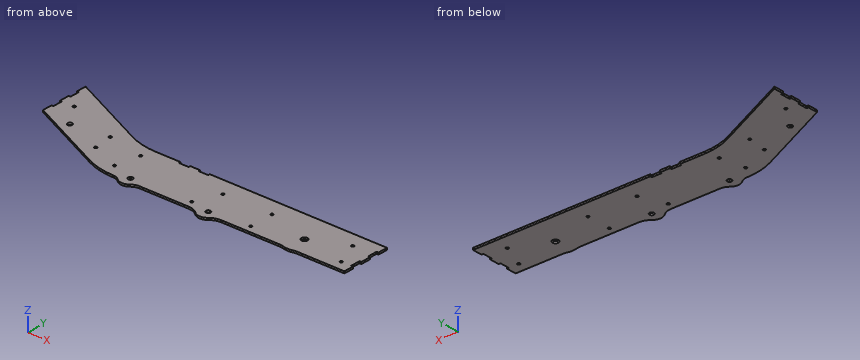
from build123d import *

# Parameters (mm, degrees)
BOSS_EXTRUDE1_DEPTH              = 4.826
SKETCH5_R                        = 3.3782
STANDOFF_HOLE_DEPTH              = 5.826
SKETCH8_W                        = 25.4
SKETCH8_H                        = 4.826
TOP_SLOTS_DEPTH                  = 5.826
BACK_AXLE_EXTENSION_DEPTH        = 4.826
LOWER_SMALL_AXLE_EXTENSION_DEPTH = 4.826
FRONT_SMALL_AXLE_EXTENSION_DEPTH = 4.826
SKETCH10_R                       = 8
SKETCH10_R_2                     = 6
NEW_AXLE_HOLES_DEPTH             = 5.826


with BuildPart() as part:
    # outer face → Boss-Extrude1 (new body)
    with BuildSketch(Plane.XY):
        with BuildLine():
            Line((622.3, 0), (24.193267589, 0))
            ThreePointArc((24.193267589, 0), (-14.28969577, 4.214569934), (-50.948259349, 16.658475465))
            Line((-50.948259349, 16.658475465), (-254, 111.343057132))
            Line((-254, 111.343057132), (-254, 136.743057132))
            Line((-254, 136.743057132), (-249.174, 136.743057132))
            Line((-249.174, 136.743057132), (-249.174, 162.143057132))
            Line((-249.174, 162.143057132), (-254, 162.143057132))
            Line((-254, 162.143057132), (-254, 187.543057132))
            Line((-254, 187.543057132), (-249.174, 187.543057132))
            Line((-249.174, 187.543057132), (-249.174, 212.943057132))
            Line((-249.174, 212.943057132), (-254, 212.943057132))
            Line((-254, 212.943057132), (-254, 238.343057132))
            Line((-254, 238.343057132), (-50.948259349, 143.658475465))
            ThreePointArc((-50.948259349, 143.658475465), (-14.28969577, 131.214569934), (24.193267589, 127))
            Line((24.193267589, 127), (622.3, 127))
            Line((622.3, 127), (622.3, 101.6))
            Line((622.3, 101.6), (617.474, 101.6))
            Line((617.474, 101.6), (617.474, 76.2))
            Line((617.474, 76.2), (622.3, 76.2))
            Line((622.3, 76.2), (622.3, 50.8))
            Line((622.3, 50.8), (617.474, 50.8))
            Line((617.474, 50.8), (617.474, 25.4))
            Line((617.474, 25.4), (622.3, 25.4))
            Line((622.3, 25.4), (622.3, 0))
        make_face()
    extrude(amount=BOSS_EXTRUDE1_DEPTH)

    # Sketch5 → standoff hole (cut, through all)
    with BuildSketch(Plane.XY.offset(4.826)):
        with Locations((-76.2, 63.5)):
            Circle(SKETCH5_R)
        with Locations((-82.55, 114.3)):
            Circle(SKETCH5_R)
        with Locations((592.074, 25.4)):
            Circle(SKETCH5_R)
        with Locations((0, 31.75)):
            Circle(SKETCH5_R)
        with Locations((211.0486, 19.05)):
            Circle(SKETCH5_R)
        with Locations((236.4486, 82.55)):
            Circle(SKETCH5_R)
        with Locations((363.4486, 82.55)):
            Circle(SKETCH5_R)
        with Locations((363.4486, 19.05)):
            Circle(SKETCH5_R)
        with Locations((566.674, 88.9)):
            Circle(SKETCH5_R)
        with Locations((12.7, 95.25)):
            Circle(SKETCH5_R)
        with Locations((-217.424, 162.143057132)):
            Circle(SKETCH5_R)
    extrude(amount=-STANDOFF_HOLE_DEPTH, mode=Mode.SUBTRACT)

    # Sketch8 → top slots (cut, through all)
    with BuildSketch(Plane.XY.offset(4.826)):
        with Locations((100.393267589, 124.587)):
            Rectangle(SKETCH8_W, SKETCH8_H)
        with Locations((151.193267589, 124.587)):
            Rectangle(SKETCH8_W, SKETCH8_H)
    extrude(amount=-TOP_SLOTS_DEPTH, mode=Mode.SUBTRACT)

    # Sketch9 → back axle extension (add)
    with BuildSketch(Plane.XY.offset(4.826)):
        with BuildLine():
            Line((498.944734517, 0), (456.603265483, 0))
            ThreePointArc((456.603265483, 0), (460.166971419, -0.251242575), (463.660176989, -1))
            ThreePointArc((463.660176989, -1), (477.774, -3), (491.887823011, -1))
            ThreePointArc((491.887823011, -1), (495.381028581, -0.251242575), (498.944734517, 0))
        make_face()
    extrude(amount=-BACK_AXLE_EXTENSION_DEPTH)

    # Sketch11 → lower small axle extension (add)
    with BuildSketch(Plane.XY.offset(4.826)):
        with BuildLine():
            Line((303.790106689, 0), (219.957893311, 0))
            ThreePointArc((219.957893311, 0), (233.396420016, -2.448688664), (245.107557324, -9.48))
            ThreePointArc((245.107557324, -9.48), (261.874, -15.8), (278.640442676, -9.48))
            ThreePointArc((278.640442676, -9.48), (290.351579984, -2.448688664), (303.790106689, 0))
        make_face()
    extrude(amount=-LOWER_SMALL_AXLE_EXTENSION_DEPTH)

    # Sketch13 → front small axle extension (add)
    with BuildSketch(Plane.XY.offset(4.826)):
        with BuildLine():
            Line((91.928424908, 0), (24.193267589, 0))
            ThreePointArc((24.193267589, 0), (33.393269649, -1.659006827), (41.434305199, -6.427034599))
            ThreePointArc((41.434305199, -6.427034599), (58.060846248, -12.625), (74.687387297, -6.427034599))
            ThreePointArc((74.687387297, -6.427034599), (82.728422848, -1.659006827), (91.928424908, 0))
        make_face()
    extrude(amount=-FRONT_SMALL_AXLE_EXTENSION_DEPTH)

    # Sketch10 → new axle holes (cut, through all)
    with BuildSketch(Plane.XY.offset(4.826)):
        with Locations((477.774, 47.8)):
            Circle(SKETCH10_R)
        with Locations((261.874, 9.6)):
            Circle(SKETCH10_R_2)
        with Locations((58.060846248, 12.775)):
            Circle(SKETCH10_R_2)
        with Locations((-176.843107922, 102.547565902)):
            Circle(SKETCH10_R_2)
    extrude(amount=-NEW_AXLE_HOLES_DEPTH, mode=Mode.SUBTRACT)


solid = part.part
Model file for the job. Use its own axes, mm. Round coordinates to 2 decimals unless told otherwise and drop trailing zeros. Order: outer loops, then holes, each group sorted by start corner. A loop starts at its lowest first (then second) coordinate and runs counter-clockwise, first axis right, second up.
(1) Band-saw the part on A-A (x = 513.5). List the corners of the cut face in (y, z), then the cut area to 3 significant figures.
(2) Drill centre lines: line 1 (Y direction, x = 303, z = 3.4); line 2 (Y direction, x = 496, z = 0.95); line 3 (Y direction, x = 0, z = 3.6). Where is each one in solid material? Low to high.
(3) Pin check, flat tips, straight feed: pin 1 (1.4 mm diameter, centred on x = -251, z = 2.5, fed in from -Y); pin 2 (4 mm diameter, centred on x = 12.7, y = 95.25, fed in from -Z); pin 3 (1 mm diameter, centred on x = 130.5, z = 2, fed in from -Y); pin 4 (1.4 mm diameter, centred on x = 620.5, z = 2.5, fed in from +Y). Stop position of each tip, or through.
(4) Band-saw the part on B-B (z = 1.45). Give the number of separate pieces and of enclosed holes in the cut face, then the cut area to 3 significant figures.
Verdict:
1. outline: (0, 0) - (127, 0) - (127, 4.83) - (0, 4.83) - close
1. area: 613 mm2
2. line 1: y = -0.01 to 127
2. line 2: y = -0.17 to 127
2. line 3: y = 1.65 to 28.37, 35.13 to 128.65
3. pin 1: stops at y = 109.62
3. pin 2: passes through
3. pin 3: stops at y = 0
3. pin 4: stops at y = 127
4. separate pieces: 1
4. enclosed holes: 15
4. area: 111,000 mm2
